from build123d import *

# Parameters (mm, degrees)
F0_W     = 16.8
F0_H     = 16.8
F0_W_2   = 12.4
F0_H_2   = 12.4
F3_DEPTH = 20
F2_W     = 16.8
F2_H     = 16.8
F2_W_2   = 13.2
F2_H_2   = 13.2
F4_DEPTH = 20
F5_R     = 1.6
F6_DEPTH = 25
F7_R     = 4.5
F8_DEPTH = 2.5
F9_SIZE  = 0.2
F10_R    = 1
F11_SIZE = 1.3


with BuildPart() as f3:
    # F0 (on Top) → F3 (new body)
    with BuildSketch(Plane.XY):
        Rectangle(F0_W, F0_H)
        Rectangle(F0_W_2, F0_H_2, mode=Mode.SUBTRACT)
    extrude(amount=F3_DEPTH)

    # F2 (on offset) → F4 (join)
    with BuildSketch(Plane.XY.offset(40)):
        Rectangle(F2_W, F2_H)
        Rectangle(F2_W_2, F2_H_2, mode=Mode.SUBTRACT)
    extrude(amount=-F4_DEPTH)

    # F5 (on face) → F6 (cut)
    with BuildSketch(Plane.YZ.offset(8.4)):
        with Locations((0, 30)):
            Circle(F5_R)
        with Locations((0, 10)):
            Circle(F5_R)
    extrude(amount=-F6_DEPTH, mode=Mode.SUBTRACT)

    # F7 (on face) → F8 (join)
    with BuildSketch(Plane(origin=(-8.4, 0, 0), x_dir=(0, -1, 0), z_dir=(-1, 0, 0))):
        with Locations((0, 10)):
            Circle(F7_R)
        Polygon((0, 13.2), (2.771281, 11.6), (2.771281, 8.4), (0, 6.8), (-2.771281, 8.4), (-2.771281, 11.6), align=None, mode=Mode.SUBTRACT)
        with Locations((0, 30)):
            Circle(F7_R)
        Polygon((0, 33.2), (2.771281, 31.6), (2.771281, 28.4), (0, 26.8), (-2.771281, 28.4), (-2.771281, 31.6), align=None, mode=Mode.SUBTRACT)
    extrude(amount=F8_DEPTH)

    # F9
    f9_edges = [f3.edges().sort_by_distance(p)[0] for p in [
        (0, 6.6, 40),
        (-6.6, 0, 40),
        (0, -6.6, 40),
        (6.6, 0, 40),
        (0, -6.2, 0),
        (6.2, 0, 0),
        (0, 6.2, 0),
        (-6.2, 0, 0),
    ]]
    chamfer(f9_edges, length=F9_SIZE)

    # F10
    f10_edges = [f3.edges().sort_by_distance(p)[0] for p in [
        (-8.4, 4.5, 10),
        (-10.9, 4.5, 10),
        (-10.9, 4.5, 30),
        (-8.4, 4.5, 30),
    ]]
    fillet(f10_edges, radius=F10_R)

    # F11
    f11_edges = [f3.edges().sort_by_distance(p)[0] for p in [
        (8.4, 8.4, 20),
        (0, 8.4, 40),
        (-8.4, 8.4, 20),
        (0, 8.4, 0),
        (-8.4, -8.4, 20),
        (0, -8.4, 40),
        (8.4, -8.4, 20),
        (0, -8.4, 0),
        (8.4, 0, 0),
        (-8.4, 0, 0),
        (-8.4, 0, 40),
        (8.4, 0, 40),
    ]]
    chamfer(f11_edges, length=F11_SIZE)


solid = f3.part
Read the model definition and answer for the solid it produces. Units are mm, in the model's axes. A direction names the side the tool comes from. Give positions to 0.01 mm unless a question says otherwise; leave off trailing zeros. Loops run counter-clockwise (first coordinate to the right, second up) from the corner with the lowest first, then second, coordinate; pieces in that order, holes last. Notation, with made-up numbers: (32.25, 29.25) -> (44.25, 29.25) arc R22 ccw to (44.25, 60.25) -> close; hole circle Ø1 at (76.5, -26.5). An arc over 180 degrees is marked (long way). Use a Markdown table: item, result.
Q1. Section B-B, the plane x = 3 is taken. Determine the outline of the cut face in (y, z).
Solved:
| item | result |
|---|---|
| outline | (-8.4, 1.3) -> (-7.1, 0) -> (-6.4, 0) -> (-6.2, 0.2) -> (-6.2, 20) -> (-6.6, 20) -> (-6.6, 39.8) -> (-6.8, 40) -> (-7.1, 40) -> (-8.4, 38.7) -> close; (6.2, 0.2) -> (6.4, 0) -> (7.1, 0) -> (8.4, 1.3) -> (8.4, 38.7) -> (7.1, 40) -> (6.8, 40) -> (6.6, 39.8) -> (6.6, 20) -> (6.2, 20) -> close |
Q2. Section A-A, the plane z = 18 is taken. Determine the outline of the cut face in (x, y).
Solved:
| item | result |
|---|---|
| outline | (-8.4, -7.1) -> (-7.1, -8.4) -> (7.1, -8.4) -> (8.4, -7.1) -> (8.4, 7.1) -> (7.1, 8.4) -> (-7.1, 8.4) -> (-8.4, 7.1) -> close; hole (-6.2, -6.2) -> (6.2, -6.2) -> (6.2, 6.2) -> (-6.2, 6.2) -> close |
Q3. Find the intervals of material crossed by line 1 along X through (y, z) = (-2, 3); line 2 along Z through (x, y) = (7.4, 0), in increasing order.
Solved:
| item | result |
|---|---|
| line 1 | x = -8.4 to -6.2, 6.2 to 8.4 |
| line 2 | z = 0.3 to 8.4, 11.6 to 28.4, 31.6 to 39.7 |
Q4. Determine the mould class of faces 1 (the face through (0, -6.6, 30)), 2 (the face through (-7.5, -7.5, 0.8)), 3 (the face through (7.513, -0.208, 31.586)) for opening direction X: pulls with the +X half, pulls with the -X half, needs draft (parallel to the pull), parting line crosses it, or undercut.
Solved:
| item | result |
|---|---|
| face 1 | undercut |
| face 2 | pulls with the -X half |
| face 3 | needs draft |
Q5. A tool of negligible diameter and unlimited length cuts with its end or side. For faces 4 (the face through (0, 6.2, 10)), 5 (the face through (0, -8.4, 20)), 6 (the face through (-9.63, -1.37, 12.41)), from which of +Z, -Z, +X, -X, +Y, -Y can it reach the whole face along a straight path? Write none if from no direction.
Solved:
| item | result |
|---|---|
| face 4 | +Z, -Z |
| face 5 | +Z, -Z, +X, -X, -Y |
| face 6 | -X |
Q6. Each of these flat-tipped pins is pushed along its axis until it touches: pin 1 (1.2 mm diameter, centred on x = -10, z = 10, fed in from +Y); pin 2 (1 mm diameter, centred on y = 5, z = 34, fed in from -X); pin 3 (1.5 mm diameter, centred on x = -7.5, z = 22, fed in from -Y); pin 4 (1.5 mm diameter, centred on x = -8, z = 15.5, fed in from +Y). Where does it stop, or does it pass through?
Solved:
| item | result |
|---|---|
| pin 1 | stops at y = 4.5 |
| pin 2 | stops at x = -8.4 |
| pin 3 | stops at y = -8.4 |
| pin 4 | stops at y = 8.25 |
